from build123d import *

# Parameters (mm, degrees)
SKETCH1_W           = 139.7
SKETCH1_H           = 18.415
BOSS_EXTRUDE1_DEPTH = 139.7


# Read off the part's stored shape, not the designer's step: Mirror2
with BuildPart() as part:
    # Sketch1 → Boss-Extrude1 (new body)
    with BuildSketch(Plane(origin=(0, 0, 0), x_dir=(1, 0, 0), z_dir=(0, 1, 0))):
        with Locations((69.85, 9.2075)):
            Rectangle(SKETCH1_W, SKETCH1_H)
    extrude(amount=BOSS_EXTRUDE1_DEPTH)

    # Sketch4 → 1/4-20 Tapped Hole1 (revolve, cut)
    with BuildSketch(Plane(origin=(139.7, 38.1, -9.2075), x_dir=(0, 0, -1), z_dir=(0, 1, 0))):
        Polygon((0, 0), (0, 20.583816902), (2.5527, 19.05), (2.5527, 0), align=None)
    revolve(axis=Axis((146.05, 38.1, -9.2075), (-1, 0, 0)), mode=Mode.SUBTRACT)

    # Sketch4 at point 2 (carried to point 2, square into its face) → 1/4-20 Tapped Hole1 at 2 (revolve, cut)
    with BuildSketch(Plane(origin=(139.7, 12.7, -9.2075), x_dir=(0, 0, -1), z_dir=(0, 1, 0))):
        Polygon((0, 0), (0, 20.583816902), (2.5527, 19.05), (2.5527, 0), align=None)
    revolve(axis=Axis((146.05, 12.7, -9.2075), (-1, 0, 0)), mode=Mode.SUBTRACT)

    # Sketch4 at point 3 (carried to point 3, square into its face) → 1/4-20 Tapped Hole1 at 3 (revolve, cut)
    with BuildSketch(Plane(origin=(69.85, 139.7, -9.2075), x_dir=(0, 0, -1), z_dir=(-1, 0, 0))):
        Polygon((0, 0), (0, 20.583816902), (2.5527, 19.05), (2.5527, 0), align=None)
    revolve(axis=Axis((69.85, 146.05, -9.2075), (0, -1, 0)), mode=Mode.SUBTRACT)

    # Sketch4 at point 4 (carried to point 4, square into its face) → 1/4-20 Tapped Hole1 at 4 (revolve, cut)
    with BuildSketch(Plane(origin=(12.7, 139.7, -9.2075), x_dir=(0, 0, -1), z_dir=(-1, 0, 0))):
        Polygon((0, 0), (0, 20.583816902), (2.5527, 19.05), (2.5527, 0), align=None)
    revolve(axis=Axis((12.7, 146.05, -9.2075), (0, -1, 0)), mode=Mode.SUBTRACT)

    # Mirror2 outline → Mirror2 (revolve, cut)
    with BuildSketch(Plane(origin=(0, 12.7, -9.2075), x_dir=(0, 1, 0), z_dir=(0, 0, -1))):
        Polygon((2.5527, 0), (2.5527, 19.05), (0, 20.583816902), (0, 0), align=None)
    revolve(axis=Axis((0, 12.7, -9.2075), (1, 0, 0)), mode=Mode.SUBTRACT)

    # Mirror2 2 outline → Mirror2 2 (revolve, cut)
    with BuildSketch(Plane(origin=(0, 38.1, -9.2075), x_dir=(0, 1, 0), z_dir=(0, 0, -1))):
        Polygon((2.5527, 0), (2.5527, 19.05), (0, 20.583816902), (0, 0), align=None)
    revolve(axis=Axis((0, 38.1, -9.2075), (1, 0, 0)), mode=Mode.SUBTRACT)

    # Mirror2 3 outline → Mirror2 3 (revolve, cut)
    with BuildSketch(Plane(origin=(127, 0, -9.2075), x_dir=(1, 0, 0), z_dir=(0, 0, 1))):
        Polygon((0, 139.7), (0, 119.116183098), (2.5527, 120.65), (2.5527, 139.7), align=None)
    revolve(axis=Axis((127, 0, -9.2075), (0, 1, 0)), mode=Mode.SUBTRACT)


solid = part.part
Here's how the part is built. I have some questions about the finished solid (model axes, mm). A direction names the side the tool comes from. Coordinates: 2 decimals unless noted, no trailing zeros.
1. For P1, Ø8, axis at y = 38.1, z = -9.21, coming from the +X side; P2, Ø4.5, axis at x = 12.7, z = -9.21, coming from the +Y side; P3, Ø4.5, axis at y = 38.1, z = -9.21, coming from the -X side; P4, Ø3, axis at y = 12.7, z = -9.21, coming from the -X side, each with a flat end and sliding along its axis, tell me the tip position at first contact or that it passes through.
2. Imagine slicing it at A-A, the plane y = 127.5. Count the separate pieces of the cut face and the enclosed holes in it, and give its area (3 significant figures).
3. For faces 4 (the cylindrical face through (130.3, 15.2, -8.7)), 5 (the cylindrical face through (10.2, 130.3, -8.7)), 6 (the cylindrical face through (9.66, 39.28, -11.47)), which set-ups out of +Z, -Z, +X, -X, +Y, -Y let a thin tool reach every point of the face, with its end or its side?
4. I need wall thicknesses on L1, parallel to Z at x = 127, y = 129 (3 decimals); L2, parallel to X at y = 134, z = -7.75; L3, parallel to Z at x = 15, y = 12 (3 decimals). Which ranges of each line are inside material? Lowest first, please.
5. If we mould it in two halves opening along Z, with no side actions, what happens to faces 1 (the flat face through (69, 69, 0)), 2 (the conical face through (70.29, 119.383, -9.15)), 3 (the flat face through (69, 0, -9))? For each: pulls with the +Z half, pulls with the -Z half, needs draft (parallel to the pull), parting line crosses it, or undercut.
Taken from the geometry:
1. P1: stops at x = 139.7
1. P2: stops at y = 120.47
1. P3: stops at x = 19.23
1. P4: stops at x = 19.68
2. separate pieces: 1
2. enclosed holes: 3
2. area: 2,510 mm2
3. face 4: +X
3. face 5: +Y
3. face 6: -X
4. L1: z = -18.415 to -11.76, -6.655 to 0
4. L2: x = 0 to 10.6, 14.8 to 67.75, 71.95 to 124.9, 129.1 to 139.7
4. L3: z = -18.415 to -11.662, -6.753 to 0
5. face 1: pulls with the +Z half
5. face 2: undercut
5. face 3: needs draft
